```python
from build123d import *

# Parameters (mm, degrees)
F0_W     = 34
F0_H     = 38
F0_W_2   = 30
F0_H_2   = 34
F1_DEPTH = 2
F2_R     = 2.875
F3_DEPTH = 7
F4_DEPTH = 2


with BuildPart() as f1:
    # F0 (on Front) → F1 (new body)
    with BuildSketch(Plane.XZ):
        Rectangle(F0_W, F0_H)
        Rectangle(F0_W_2, F0_H_2, mode=Mode.SUBTRACT)
        Rectangle(F0_W_2, F0_H_2)
    extrude(amount=F1_DEPTH)

    # F2 (on Front) → F3 (join)
    with BuildSketch(Plane.XZ):
        Circle(F2_R)
    extrude(amount=F3_DEPTH)

    # F0 (on Front) → F4 (join)
    with BuildSketch(Plane.XZ):
        Rectangle(F0_W, F0_H)
        Rectangle(F0_W_2, F0_H_2, mode=Mode.SUBTRACT)
    extrude(amount=-F4_DEPTH)


solid = f1.part
```
Model file for the job. Use its own axes, mm. A direction names the side the tool comes from. Give positions to 0.01 mm unless a question says otherwise; leave off trailing zeros. Order: outer loops, then holes, each group sorted by start corner. A loop starts at its lowest first (then second) coordinate and runs counter-clockwise, first axis right, second up.
1) Saw through at C-C, the plane z = -12.5. Write the cut outline in (x, y).
2) Wall check: probe 1 along X at (y, z) = (0.5, 8); probe 2 along Z at (x, y) = (-14.5, 1); probe 3 along Y at (x, z) = (11, 6). Give the ranges that are in metal, low to high.
3) Saw through at B-B, the plane x = 0. Write the cut outline in (y, z) (3 decimals), then the cut area to 3 significant figures.
4) Saw through at A-A, the plane y = 0.5. Write the cut outline in (x, z), then the cut area to 3 significant figures.
5) Mould opens along X. For faces 4 (the flat face through (0, 1, 17)), 5 (the flat face through (0, -7, 0)), 6 (the flat face through (17, 0, 0)) say: +X half, -X half, draft (parallel to the pull), parting line (faces both ways), or undercut.
6) Pin check, flat tip, straight feed: pin 1 (10 mm diameter, centred on x = 1.5, z = 11, fed in from +Y). Stop position of the tip, or through.
7) Saw through at D-D, the plane z = 0. Write the cut outline in (x, y) (3 decimals).
8) 3-axis set-ups, long thin cutter, end or side, ignore diameter. For faces 1 (the flat face through (0, 0, 0)), 2 (the flat face through (-17, 0, 0)), 3 (the cylindrical face through (-0.37, -4.46, 2.85)): which of +Z, -Z, +X, -X, +Y, -Y reach the whole face in a straight line?
Computed:
1. outline: (-17, -2) - (17, -2) - (17, 2) - (15, 2) - (15, 0) - (-15, 0) - (-15, 2) - (-17, 2) - close
2. probe 1: x = -17 to -15, 15 to 17
2. probe 2: z = -19 to -17, 17 to 19
2. probe 3: y = -2 to 0
3. outline: (-7, -2.875) - (-2, -2.875) - (-2, -19) - (2, -19) - (2, -17) - (0, -17) - (0, 17) - (2, 17) - (2, 19) - (-2, 19) - (-2, 2.875) - (-7, 2.875) - close
3. area: 113 mm2
4. outline: (-17, -19) - (17, -19) - (17, 19) - (-17, 19) - close; hole (-15, -17) - (15, -17) - (15, 17) - (-15, 17) - close
4. area: 272 mm2
5. face 4: undercut
5. face 5: draft
5. face 6: +X half
6. pin 1: stops at y = 0
7. outline: (-17, -2) - (-2.875, -2) - (-2.875, -7) - (2.875, -7) - (2.875, -2) - (17, -2) - (17, 2) - (15, 2) - (15, 0) - (-15, 0) - (-15, 2) - (-17, 2) - close
8. face 1: +Y
8. face 2: +Z, -Z, -X, +Y, -Y
8. face 3: -Y
